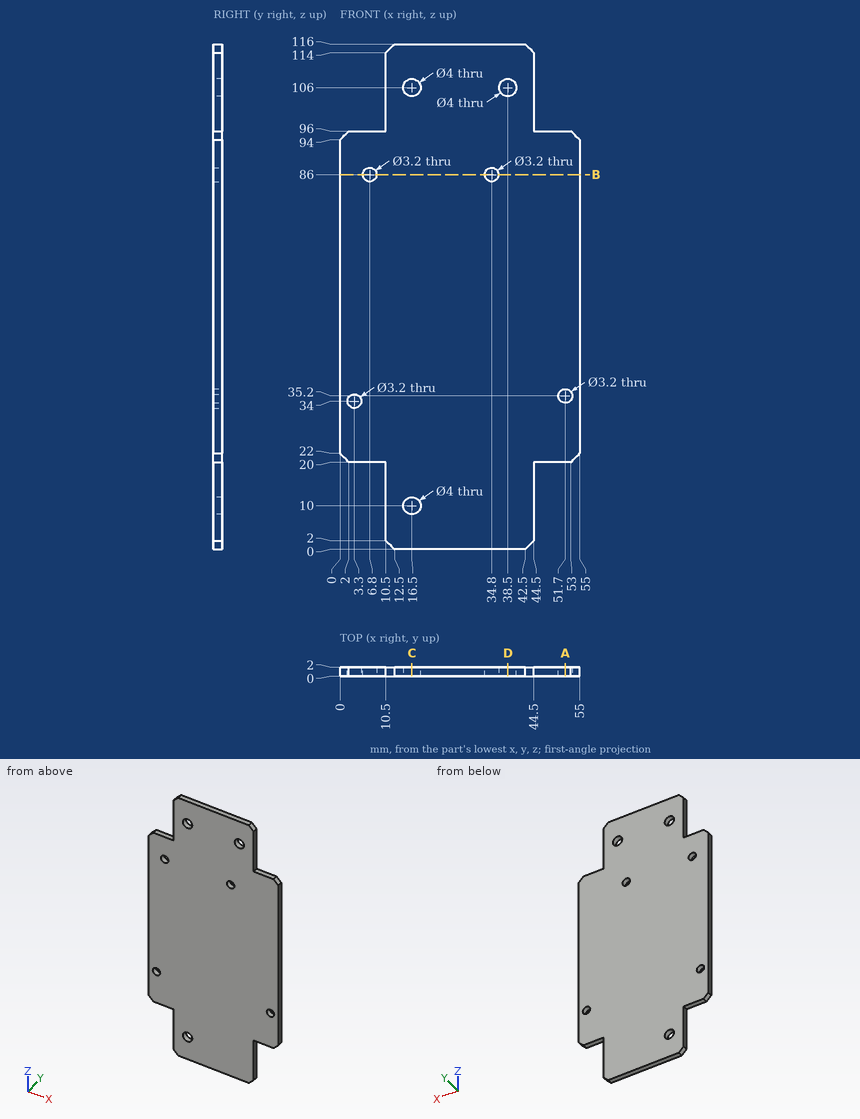
Geometry check sheet. Reference: drawing and pictorial views, mm from the part's lowest x, y, z. Round coordinates to 2 decimals unless told otherwise and drop trailing zeros. Loops run counter-clockwise (first coordinate to the right, second up) from the corner with the lowest first, then second, coordinate; pieces in that order, holes last. Notation, with made-up numbers: (78, 76) -> (112, 76) arc R19 cw to (112, 80) -> close; hole circle Ø3 at (-38.5, -12.75). An arc over 180 degrees is marked (long way). Use a Markdown table: item, result.
(1) Sectioned sample at B-B (z = 86). Enter the section's corners in (x, y).
Calculated:
| item | result |
|---|---|
| outline | (0, 0) -> (5.2, 0) -> (5.2, 2) -> (0, 2) -> close; (8.4, 0) -> (33.2, 0) -> (33.2, 2) -> (8.4, 2) -> close; (36.4, 0) -> (55, 0) -> (55, 2) -> (36.4, 2) -> close |
(2) Sectioned sample at D-D (x = 38.5). Enter the section's corners in (y, z), then the cut area to 3 significant figures.
Calculated:
| item | result |
|---|---|
| outline | (0, 0) -> (2, 0) -> (2, 104) -> (0, 104) -> close; (0, 108) -> (2, 108) -> (2, 116) -> (0, 116) -> close |
| area | 224 mm² |
(3) Sectioned sample at C-C (x = 16.5). Enter the section's corners in (y, z), then the cut area to 3 significant figures.
Calculated:
| item | result |
|---|---|
| outline | (0, 0) -> (2, 0) -> (2, 8) -> (0, 8) -> close; (0, 12) -> (2, 12) -> (2, 104) -> (0, 104) -> close; (0, 108) -> (2, 108) -> (2, 116) -> (0, 116) -> close |
| area | 216 mm² |
(4) Scan lines: probe 1 along X at (y, z) = (1.35, 106); probe 2 along Z at (x, y) = (16.5, 1.4); probe 3 along X at (y, z) = (1, 86). Record each from-to range of solid material in increasing order.
Calculated:
| item | result |
|---|---|
| probe 1 | 10.5 to 14.5, 18.5 to 36.5, 40.5 to 44.5 |
| probe 2 | 0 to 8, 12 to 104, 108 to 116 |
| probe 3 | 0 to 5.2, 8.4 to 33.2, 36.4 to 55 |
(5) Sectioned sample at A-A (x = 51.7). Enter the section's corners in (y, z), then the cut area to 3 significant figures.
Calculated:
| item | result |
|---|---|
| outline | (0, 20) -> (2, 20) -> (2, 33.6) -> (0, 33.6) -> close; (0, 36.8) -> (2, 36.8) -> (2, 96) -> (0, 96) -> close |
| area | 146 mm² |
(6) Go/stop test with flat-tipped pins: P1, Ø0.6, axis at y = 1, z = 8, coming from the -X side; P2, Ø0.6, axis at x = 49, y = 1, coming from the -Z side. Record where each tip stops, or that it passes through.
Calculated:
| item | result |
|---|---|
| P1 | x = 10.5 |
| P2 | z = 20 |
